Autodesk Inventor part; units mm, degrees
ref_plane "Start Plane" through (0, 0, -15) normal (0, 0, 1) x (1, 0, 0)
ref_plane "End Plane" through (0, 0, 486) normal (0, 0, 1) x (1, 0, 0)
ref_plane "Work Plane4" through (-15, 0, -15) normal (0.7071, 0, -0.7071) x (-0.7071, 0, -0.7071)
ref_plane "Start Plane" through (0, 0, -15) normal (0, 0, 1) x (1, 0, 0)
ref_plane "End Plane" through (0, 0, 486) normal (0, 0, 1) x (1, 0, 0)
sketch "Sketch" plane through (0, 0, 0) normal (0, 0, 1) x (1, 0, 0)
  line L0 (-15, -9) -> (-15, 9)
  line L1 (-9, 15) -> (9, 15)
  line L2 (15, 9) -> (15, -9)
  line L3 (9, -15) -> (-9, -15)
  arc A0 (-15, -9) -> (-9, -15) centre (-9, -9) ccw
  arc A1 (-9, 15) -> (-15, 9) centre (-9, 9) ccw
  arc A2 (15, 9) -> (9, 15) centre (9, 9) ccw
  arc A3 (9, -15) -> (15, -9) centre (9, -9) ccw
  arc A4 (-9, 12) -> (-12, 9) centre (-9, 9) ccw
  line L4 (-9, 12) -> (9, 12)
  arc A5 (12, 9) -> (9, 12) centre (9, 9) ccw
  line L5 (12, 9) -> (12, -9)
  arc A6 (9, -12) -> (12, -9) centre (9, -9) ccw
  line L6 (9, -12) -> (-9, -12)
  arc A7 (-12, -9) -> (-9, -12) centre (-9, -9) ccw
  line L7 (-12, -9) -> (-12, 9)
  line L8 (0, 22.7397) -> (0, -22.7397) construction
  line L9 (-22.7397, 0) -> (22.7397, 0) construction
  dimension "d7" = 6
  dimension "d10" = 30
  dimension "d11" = 30
  dimension "d12" = 3
  dimension "d15" = 15
  dimension "d16" = 15
extrude "Body" add sketch "Sketch" along normal up to surface (501 mm away) from surface at -15
sketch "Sketch3" plane through (0, 0, 0) normal (0, 0, 1) x (1, 0, 0)
  line L0 (0, 0) -> (10, 0)
ref_plane "Work Plane3" through (0, 0, 0) normal (0, -1, 0) x (1, 0, 0)
ref_plane "Work Plane4" through (-15, 0, -15) normal (0.7071, 0, -0.7071) x (-0.7071, 0, -0.7071)
split "Split1" plane through (-15, 0, -15) removes the side toward (0.7071, 0, -0.7071)
sketch "Sketch4" plane through (0, 0, 0) normal (0, -1, 0) x (1, 0, 0)
  line L0 (-2, -15) -> (12, -15)
  line L1 (-2, 486) -> (12, 486)
  dimension "d18" = 501
equation "\"d7\" = G_IR"
equation "\"d10\" = G_H"
equation "\"d11\" = G_W"
equation "\"d12\" = G_T"
equation "\"d15\" = 0.5 * d10"
equation "\"d16\" = 0.5 * d11"
equation "\"d3\" = G_L"
equation "\"G_W\" = 30"
equation "\"G_H\" = 30"
equation "\"G_T\" = 3"
equation "\"G_IR\" = 6"
equation "\"G_L\" = d18"
equation "\"G_OFFSET_START\" = 15.00001"
equation "\"G_OFFSET_END\" = 0"
equation "\"d13\" = -G_OFFSET_START"
equation "\"d14\" = G_OFFSET_END + B_L"
equation "\"B_L\" = 485.99998"
properties part number "DIN EN 10219-2 - 30 x 30 x 3  - 501" material "Steel, Mild"
Geometry check sheet. Reference: the model listing, model coordinates, mm. A direction names the side the tool comes from. Give positions to 0.01 mm unless a question says otherwise; leave off trailing zeros. Write each loop counter-clockwise with the first axis right and the second up, starting at its lowest first coordinate (ties: lowest second). Pieces come first, ordered by that corner, then holes.
1) Set-up check for faces 1 (the face through (15, 0, 247)), 2 (the face through (-12, 0, 234)): record each of +Z, -Z, +X, -X, +Y, -Y from which the full face is reachable in a straight line by a thin tool's end or side.
Values follow:
face 1: +Z, -Z, +X, +Y, -Y
face 2: +Z, -Z
2) Go/stop test with a flat-tipped pin: pin 1 Ø8 at (x, y) = (-7, 10.5) entering from -Z. Record where the tip stops, or that it passes through.
Values follow:
pin 1: stops at z = -10.92
3) Cross-section at B-B (y = 0). Record the boundary of the cut face in (x, z), plus the area to 3 significant figures.
Values follow:
outline: (-15, -15) - (-12, -12) - (-12, 486) - (-15, 486) - close; (12, 12) - (15, 15) - (15, 486) - (12, 486) - close
area: 2,920 mm2
4) Thickness scan on line 1 (Y direction, x = 8, z = 278); line 2 (X direction, y = 7, z = 6.5). Record the ranges inside material, lowest first.
Values follow:
line 1: y = -15 to -12, 12 to 15
line 2: x = -15 to -12
5) Cross-section at A-A (x = -4.75). Record the boundary of the cut face in (y, z), plus the area to 3 significant figures.
Values follow:
outline: (-15, -4.75) - (-12, -4.75) - (-12, 486) - (-15, 486) - close; (12, -4.75) - (15, -4.75) - (15, 486) - (12, 486) - close
area: 2,940 mm2
6) Release check for a two-part mould opening along Y. For faces 3 (the face through (-12.3, 0.1, 486)), 4 (the face through (0, -12, 235)), 5 (the face through (0, -15, 235)) record: released by +Y, released by -Y, zero draft, split by the parting line, or undercut.
Values follow:
face 3: zero draft
face 4: undercut
face 5: released by -Y
7) Cross-section at C-C (z = 249.5). Record the boundary of the cut face in (x, y).
Values follow:
outline: (-15, -9) arc R6 ccw to (-9, -15) - (9, -15) arc R6 ccw to (15, -9) - (15, 9) arc R6 ccw to (9, 15) - (-9, 15) arc R6 ccw to (-15, 9) - close; hole (-12, -9) arc R3 ccw to (-9, -12) - (9, -12) arc R3 ccw to (12, -9) - (12, 9) arc R3 ccw to (9, 12) - (-9, 12) arc R3 ccw to (-12, 9) - close
